from build123d import *

# Parameters (mm, degrees)
F1_DEPTH = 25
F2_R     = 4.99999


# Not quite as in the source:
# - a fillet or chamfer is up to 0.001 mm smaller than in the source, because OpenCascade refuses the exact size


with BuildPart() as f1:
    # F0 (on Top) → F1 (new body)
    with BuildSketch(Plane.XY):
        with BuildLine():
            Line((-4.1666666667, 24.6503324296), (-62.5, 14.7901994577))
            ThreePointArc((-62.5, 14.7901994577), (-75, 0), (-62.5, -14.7901994577))
            Line((-62.5, -14.7901994577), (-4.1666666667, -24.6503324296))
            ThreePointArc((-4.1666666667, -24.6503324296), (25, 0), (-4.1666666667, 24.6503324296))
        make_face()
        with BuildLine():
            ThreePointArc((-60.8333333333, -4.9300664859), (-65, 0), (-60.8333333333, 4.9300664859))
            Line((-60.8333333333, 4.9300664859), (-2.5, 14.7901994577))
            ThreePointArc((-2.5, 14.7901994577), (15, 0), (-2.5, -14.7901994577))
            Line((-2.5, -14.7901994577), (-60.8333333333, -4.9300664859))
        make_face(mode=Mode.SUBTRACT)
    extrude(amount=F1_DEPTH)

    # F2 (radius 5 in the source; OpenCascade refuses exactly that, so slightly less here)
    f2_edges = [f1.edges().sort_by_distance(p)[0] for p in [
        (25, 0, 25),
        (-33.333333, 19.720266, 25),
        (-75, 0, 25),
        (-33.333333, -19.720266, 25),
        (-31.666667, 9.860133, 25),
        (15, 0, 25),
        (-31.666667, -9.860133, 25),
        (-65, 0, 25),
        (-4.166667, -24.650332, 12.5),
        (-4.166667, 24.650332, 12.5),
        (25, 0, 0),
    ]]
    fillet(f2_edges, radius=F2_R)


solid = f1.part
Work out the finished part from the listing and answer in its coordinate system (mm). A direction names the side the tool comes from. Give positions to 0.01 mm unless a question says otherwise; leave off trailing zeros. Loops run counter-clockwise (first coordinate to the right, second up) from the corner with the lowest first, then second, coordinate; pieces in that order, holes last. Notation, with made-up numbers: (-35.5, -30) -> (-4.5, -30) arc R24 ccw to (-4.5, 4) -> close; hole circle Ø1 at (58.5, 59). An arc over 180 degrees is marked (long way). Use a Markdown table: item, result. Add a question column.
1. Flat-ended cylindrical pins translate along their axes: pin 1 Ø1 at (x, z) = (-49, 9) entering from -Y; pin 2 Ø10 at (x, y) = (-64, 16.5) entering from +Z; pin 3 Ø5 at (x, y) = (-64.5, 14.5) entering from +Z. Find the tip coordinate at first contact, or state that the pin passes through.
2. For faces 5 (the cylindrical face through (-32.69, -18.38, 1.5)), 6 (the flat face through (-31.26, -9.93, 9.86)), 7 (the cylindrical face through (-31.5, 11.34, 23.5)), determine the directions among +Z, -Z, +X, -X, +Y, -Y from which every point of the face is accessible in a straight line to the end or side of a thin tool.
3. Determine the mould class of faces 1 (the cylindrical face through (-75, 0, 12)), 2 (the cylindrical face through (-32.3, -11.2, 23.5)), 3 (the flat face through (-22, -12, 0)), 4 (the cylindrical face through (-33.504, 18.245, 23.496)) for opening direction Y: released by +Y, released by -Y, zero draft, split by the parting line, or undercut.
4. Section B-B on z = 18.5 is taken. Determine the outline of the cut face in (x, y), and give its area (3 significant figures).
5. Find the intervals of material crossed by probe 1 along Y at (x, z) = (0, 14.25); probe 2 along Y at (x, z) = (-29.5, 9.25); probe 3 along X at (y, z) = (-4, 10.75), in increasing order.
Results below:
| question | item | result |
|---|---|---|
| 1 | pin 1 | stops at y = -17.16 |
| 1 | pin 2 | stops at z = 24.59 |
| 1 | pin 3 | stops at z = 24.22 |
| 2 | face 5 | -Z, -X, -Y |
| 2 | face 6 | +Z, -Z |
| 2 | face 7 | +Z |
| 3 | face 1 | split by the parting line |
| 3 | face 2 | undercut |
| 3 | face 3 | zero draft |
| 3 | face 4 | released by +Y |
| 4 | outline | (-62.5, -14.79) -> (-4.17, -24.65) arc R25 ccw (long way) to (-4.17, 24.65) -> (-62.5, 14.79) arc R15 ccw to start; hole (-60.83, -4.93) -> (-2.5, -14.79) arc R15 ccw (long way) to (-2.5, 14.79) -> (-60.83, 4.93) arc R5 ccw to start |
| 4 | area | 2,160 mm^2 |
| 5 | probe 1 | y = -25 to -15, 15 to 25 |
| 5 | probe 2 | y = -20.37 to -10.23, 10.23 to 20.37 |
| 5 | probe 3 | x = -74.46 to -63, 14.46 to 24.68 |
